Can you work these out from the model? Positions are in its coordinate system, mm. Face numbers are marked on the shaded views. A direction names the side the tool comes from. Give positions to 0.01 mm unless a question says otherwise; leave off trailing zeros. Write each loop counter-clockwise with the first axis right and the second up, starting at its lowest first coordinate (ties: lowest second). Pieces come first, ordered by that corner, then holes.
1. Suppose I cut it at C-C (x = 0.5). Please give me the cut outline in (y, z).
2. I'm going to push flat-ended pins straight in: pin 1 (1.5 mm diameter, centred on x = 3.5, z = -6, fed in from -Y); pin 2 (0.9 mm diameter, centred on x = 2.5, y = 9, fed in from -Z); pin 3 (1.3 mm diameter, centred on x = 1.5, z = 1.5, fed in from -Y). Where does each tip first touch, or does it pass through?
3. If I drill on probe 1 along Y at (x, z) = (4.25, -2); probe 2 along Z at (x, y) = (1.85, 1.75); probe 3 along Z at (x, y) = (0.2, 0.75), over which ranges is the centre line in solid material (lowest first)?
4. Suppose I cut it at D-D (z = -6.25). Please give me the cut outline in (x, y), and give its area (3 significant figures).
5. Suppose I cut it at A-A (z = -2.25). Please give me the cut outline in (x, y), and give its area (3 significant figures).
6. Thinking about a two-plate mould opening in Z: for the marked faces 4, 5, 6 and 7, which applies, pulls with the +Z half, pulls with the -Z half, needs draft (parallel to the pull), parting line crosses it, or undercut?
7. On a 3-axis mill with a long thin cutter (end or side, diameter ignored), from which of +Z, -Z, +X, -X, +Y, -Y can I reach the whole of each face in a straight line? I mean the marked faces 1, 2 and 3. Say none if no direction works.
8. Suppose I cut it at B-B (y = 0). Please give me the cut outline in (x, z), and give its area (3 significant figures).
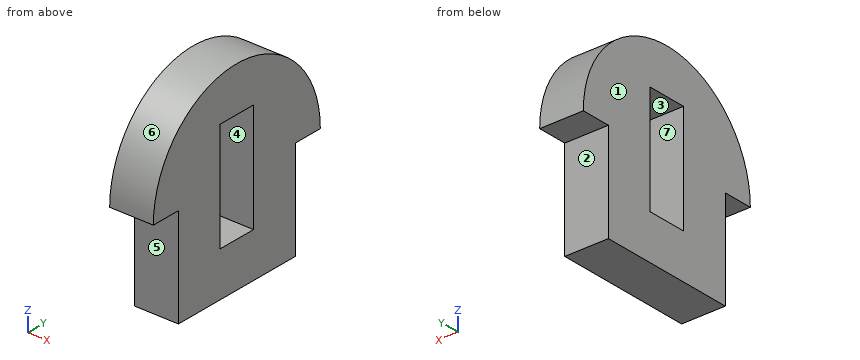
```python
from build123d import *

# Parameters (mm, degrees)
SKETCH1_W           = 11
SKETCH1_H           = 4
BOSS_EXTRUDE1_DEPTH = 4.4


with BuildPart() as part:
    # Sketch1 → Boss-Extrude1 (new body)
    with BuildSketch(Plane(origin=(0, 0, 0), x_dir=(0, 0, -1), z_dir=(1, 0, 0))):
        with BuildLine():
            Line((0, 10), (0, 7))
            Line((0, 7), (10, 7))
            Line((10, 7), (10, -7))
            Line((10, -7), (0, -7))
            Line((0, -7), (0, -10))
            ThreePointArc((0, -10), (-10, 0), (0, 10))
        make_face()
        Rectangle(SKETCH1_W, SKETCH1_H, mode=Mode.SUBTRACT)
    extrude(amount=BOSS_EXTRUDE1_DEPTH)


solid = part.part
```
Checks:
1. outline: (-10, 0) - (-7, 0) - (-7, -10) - (7, -10) - (7, 0) - (10, 0) arc R10 ccw to start; hole (-2, -5.5) - (2, -5.5) - (2, 5.5) - (-2, 5.5) - close
2. pin 1: stops at y = -7
2. pin 2: stops at z = 0
2. pin 3: stops at y = -9.96
3. probe 1: y = -7 to -2, 2 to 7
3. probe 2: z = -10 to -5.5, 5.5 to 9.85
3. probe 3: z = -10 to -5.5, 5.5 to 9.97
4. outline: (0, -7) - (4.4, -7) - (4.4, 7) - (0, 7) - close
4. area: 61.6 mm2
5. outline: (0, -7) - (4.4, -7) - (4.4, -2) - (0, -2) - close; (0, 2) - (4.4, 2) - (4.4, 7) - (0, 7) - close
5. area: 44.0 mm2
6. face 4: undercut
6. face 5: needs draft
6. face 6: pulls with the +Z half
6. face 7: undercut
7. face 1: +Z, -Z, -X, +Y, -Y
7. face 2: -Z, +X, -X, +Y
7. face 3: +X, -X
8. outline: (0, -10) - (4.4, -10) - (4.4, -5.5) - (0, -5.5) - close; (0, 5.5) - (4.4, 5.5) - (4.4, 10) - (0, 10) - close
8. area: 39.6 mm2
